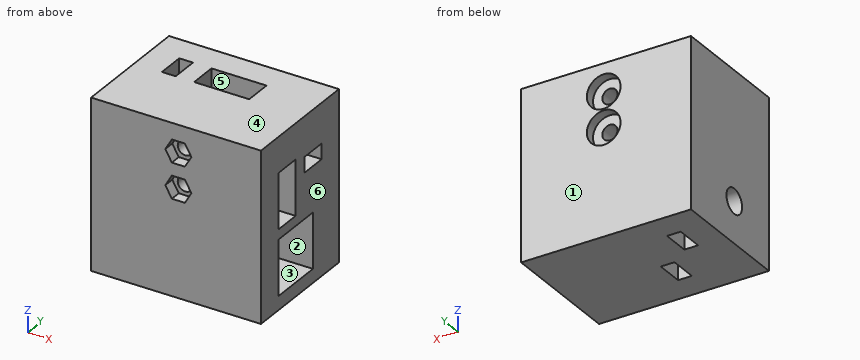
from build123d import *

# Parameters (mm, degrees)
MAIN_BLOCK_DEPTH                        = 45
BOTTOM_IDLER_CUTOUT_DEPTH               = 10
TOP_IDLER_CUTOUT_DEPTH                  = 10
BELT_PASSTHROUGH_SKETCH_W               = 5
BELT_PASSTHROUGH_SKETCH_H               = 61.4
BELT_PASSTHROUGH_DEPTH                  = 10
F_2020VSLOTCUTOUTSKETCH_W               = 20
F_2020VSLOTCUTOUTSKETCH_H               = 20
EXTRUSIONMOUNTINGSLOT_DEPTH             = 20
CBORE_FOR_M5_HEX_HEAD_BOLT1_D           = 5.5
CBORE_FOR_M5_HEX_HEAD_BOLT1_CBORE_D     = 12.24
CBORE_FOR_M5_HEX_HEAD_BOLT1_CBORE_DEPTH = 3.58
NUTTRAPS_DEPTH                          = 4
EXTRUSIONMOUNTINGCOUNTERBORESKETCH_R    = 4.5
EXTRUSIONMOUNTINGCOUNTERBORE_DEPTH      = 31.7
EXTRUSIONMOUNTINGHOLESKETCH_R           = 2.65
EXTRUSIONMOUNTINGHOLE_DEPTH             = 66.991287304


with BuildPart() as part:
    # MainBlockSketch → Main Block (new body)
    with BuildSketch(Plane(origin=(0, 0, 0), x_dir=(1, 0, 0), z_dir=(0, 1, 0))):
        Polygon((-41.7, -36.4), (20, -36.4), (20, -20), (20, -15), (20, 0), (20, 20), (20, 25), (-41.7, 25), (-41.7, 20), (-41.7, -15), align=None)
    extrude(amount=MAIN_BLOCK_DEPTH)

    # Bottom Idler Cutout Sketch → Bottom Idler Cutout (cut)
    with BuildSketch(Plane(origin=(0, 10, 0), x_dir=(1, 0, 0), z_dir=(0, 1, 0))):
        with BuildLine():
            Line((-10, -23.6), (20, -23.6))
            Line((20, -23.6), (20, -3.6))
            Line((20, -3.6), (-10, -3.6))
            ThreePointArc((-10, -3.6), (-12.588190451, -3.940741737), (-15, -4.939745962))
            Line((-15, -4.939745962), (-15, 25))
            Line((-15, 25), (-20, 25))
            Line((-20, 25), (-20, -13.6))
            ThreePointArc((-20, -13.6), (-17.071067812, -20.671067812), (-10, -23.6))
        make_face()
    extrude(amount=BOTTOM_IDLER_CUTOUT_DEPTH, mode=Mode.SUBTRACT)

    # Top Idler Cutout Sketch → Top Idler Cutout (cut)
    with BuildSketch(Plane(origin=(0, 25, 0), x_dir=(1, 0, 0), z_dir=(0, 1, 0))):
        with BuildLine():
            Line((-20, -26.4), (-20, -36.4))
            Line((-20, -36.4), (0, -36.4))
            Line((0, -36.4), (0, -26.4))
            ThreePointArc((0, -26.4), (-0.258342613, -24.141657387), (-1.020022272, -22))
            Line((-1.020022272, -22), (20, -22))
            Line((20, -22), (20, -16.4))
            Line((20, -16.4), (-10, -16.4))
            ThreePointArc((-10, -16.4), (-17.071067812, -19.328932188), (-20, -26.4))
        make_face()
    extrude(amount=TOP_IDLER_CUTOUT_DEPTH, mode=Mode.SUBTRACT)

    # Belt Passthrough Sketch → Belt Passthrough (cut)
    with BuildSketch(Plane(origin=(0, 25, 0), x_dir=(1, 0, 0), z_dir=(0, 1, 0))):
        with Locations((-29.2, -5.7)):
            Rectangle(BELT_PASSTHROUGH_SKETCH_W, BELT_PASSTHROUGH_SKETCH_H)
    extrude(amount=BELT_PASSTHROUGH_DEPTH, mode=Mode.SUBTRACT)

    # 2020VSlotCutoutSketch → ExtrusionMountingSlot (cut)
    with BuildSketch(Plane(origin=(0, 10, 0), x_dir=(1, 0, 0), z_dir=(0, 1, 0))):
        with Locations((10, 10)):
            Rectangle(F_2020VSLOTCUTOUTSKETCH_W, F_2020VSLOTCUTOUTSKETCH_H)
    extrude(amount=EXTRUSIONMOUNTINGSLOT_DEPTH, mode=Mode.SUBTRACT)

    # CBORE for M5 Hex Head Bolt1 (through all)
    with Locations(Plane(origin=(0, 45, 0), x_dir=(1, 0, 0), z_dir=(0, 1, 0))):
        with Locations((-10, -26.4), (-10, -13.6)):
            CounterBoreHole(CBORE_FOR_M5_HEX_HEAD_BOLT1_D / 2, CBORE_FOR_M5_HEX_HEAD_BOLT1_CBORE_D / 2, CBORE_FOR_M5_HEX_HEAD_BOLT1_CBORE_DEPTH)

    # Nut Trap Sketch → NutTraps (cut)
    with BuildSketch(Plane(origin=(0, 0, 0), x_dir=(1, 0, 0), z_dir=(0, 1, 0))):
        Polygon((-7.632863896, -9.5), (-12.367136104, -9.5), (-14.734272207, -13.6), (-12.367136104, -17.7), (-7.632863896, -17.7), (-5.265727793, -13.6), align=None)
        Polygon((-7.632863896, -22.3), (-12.367136104, -22.3), (-14.734272207, -26.4), (-12.367136104, -30.5), (-7.632863896, -30.5), (-5.265727793, -26.4), align=None)
    extrude(amount=NUTTRAPS_DEPTH, mode=Mode.SUBTRACT)

    # ExtrusionMountingCounterBoreSketch → ExtrusionMountingCounterbore (cut)
    with BuildSketch(Plane(origin=(-41.7, 0, 0), x_dir=(0, 0, -1), z_dir=(1, 0, 0))):
        with Locations(Location((10, 20, 0), (0, 0, 180))):
            Circle(EXTRUSIONMOUNTINGCOUNTERBORESKETCH_R)
    extrude(amount=EXTRUSIONMOUNTINGCOUNTERBORE_DEPTH, mode=Mode.SUBTRACT)

    # ExtrusionMountingHoleSketch → extrusionMountingHole (cut, through all)
    with BuildSketch(Plane.ZY.offset(10)):
        with Locations((-10, 20)):
            Circle(EXTRUSIONMOUNTINGHOLESKETCH_R)
    extrude(amount=-EXTRUSIONMOUNTINGHOLE_DEPTH, mode=Mode.SUBTRACT)


solid = part.part
Design review of the part built by this model. Coordinates are the model's own, in mm. Face numbers are marked on the shaded views. A direction names the side the tool comes from. Give positions to 0.01 mm unless a question says otherwise; leave off trailing zeros. Loops run counter-clockwise (first coordinate to the right, second up) from the corner with the lowest first, then second, coordinate; pieces in that order, holes last. Notation, with made-up numbers: M 26.5,51.25 L 57.5,51.25 A16 cw 57.5,78.25 Z; hole C 24.25,7.25 d2. An arc over 180 degrees is marked long. Write item = value, one per line.
Q1. We need section A-A (z = -10). Give the boundary of the cut face in (x, y).
Output values:
outline = M -41.7,0 L 20,0 L 20,10 L 0,10 L 0,17.35 L -10,17.35 L -10,15.5 L -15,15.5 L -15,10 L -20,10 L -20,15.5 L -41.7,15.5 Z; M -41.7,24.5 L -10,24.5 L -10,22.65 L 0,22.65 L 0,30 L 20,30 L 20,45 L -41.7,45 Z; hole M -31.7,25 L -26.7,25 L -26.7,35 L -31.7,35 Z
Q2. We need section C-C (x = 8). Give the boundary of the cut face in (y, z), plus the area to 3 significant figures.
Output values:
outline = M 0,-25 L 45,-25 L 45,36.4 L 0,36.4 Z; hole M 10,-20 L 30,-20 L 30,0 L 10,0 Z; hole M 10,3.6 L 20,3.6 L 20,23.6 L 10,23.6 Z; hole M 25,16.4 L 35,16.4 L 35,22 L 25,22 Z
area = 2,110 mm^2
Q3. To check wall thickness, follow line 1 (Z direction, x = -10, y = 6.7); line 2 (Z direction, x = -10, y = 43.9); line 3 (Y direction, x = -15, z = 20.5). State the ranges of each line that lie inside material, in increasing order. Write a range as [from, to].
Output values:
line_1 = [-25, 10.85], [16.35, 23.65], [29.15, 36.4]
line_2 = [-25, 7.48], [19.72, 20.28], [32.52, 36.4]
line_3 = [0, 10], [20, 25], [35, 45]
Q4. We need section D-D (z = 2). Give the boundary of the cut face in (x, y).
Output values:
outline = M -41.7,0 L 20,0 L 20,45 L -41.7,45 Z; hole M -31.7,25 L -26.7,25 L -26.7,35 L -31.7,35 Z; hole M -20,10 L -15,10 L -15,20 L -20,20 Z
Q5. We need section B-B (y = 12). Give the boundary of the cut face in (x, z).
Output values:
outline = M -41.7,-25 L -20,-25 L -20,13.6 A10 cw -10,23.6 L 20,23.6 L 20,36.4 L -41.7,36.4 Z; M -15,-25 L 20,-25 L 20,-20 L 0,-20 L 0,0 L 20,0 L 20,3.6 L -10,3.6 A10 cw -15,4.94 Z; hole C -10,26.4 d5.5
Q6. Insertion check: pin 1 (3 mm diameter, centred on x = -13, y = 31.5, fed in from +Z); pin 2 (6 mm diameter, centred on x = -11, z = 28.5, fed in from +Y). Each pin has a flat end and moves straight along its axis. Give the tip position at first contact, or say it passes through.
Output values:
pin_1 = 17.47
pin_2 = 41.42
Q7. For the marked faces 5 and 6, list the 3-axis set-ups (+Z, -Z, +X, -X, +Y, -Y) from which the entire face can be reached by the end or side of a thin tool; tool diameter is ignored.
Output values:
face_5 = none
face_6 = +Z, -Z, +X, +Y, -Y
Q8. Draft analysis for pull direction Y (two halves, no side actions). For the marked faces 1, 2, 3 and 4, state which applies: +Y half, -Y half, draft (parallel to the pull), parting line (faces both ways), or undercut.
Output values:
face_1 = +Y half
face_2 = undercut
face_3 = undercut
face_4 = draft
